from build123d import *

# Parameters (mm, degrees)
F1_DEPTH = 121.92
F3_DEPTH = 60.96
F4_W     = 60.96
F4_H     = 40.64
F5_DEPTH = 121.921


with BuildPart() as f1:
    # F0 (on Front) → F1 (new body)
    with BuildSketch(Plane.XZ):
        Polygon((137.16, -40.64), (137.16, 40.64), (15.24, 40.64), (-137.16, 40.64), (-137.16, -40.64), align=None)
        Polygon((15.24, 40.64), (137.16, 40.64), (137.16, 101.6), (106.68, 101.6), (106.68, 121.92), (45.72, 121.92), (45.72, 101.6), (15.24, 101.6), align=None)
    extrude(amount=F1_DEPTH)

    # F2 (on face) → F3 (cut)
    with BuildSketch(Plane.XY.offset(40.64)):
        Polygon((15.24, -91.111548), (15.24, -30.151548), (-45.72, -30.151548), (-106.68, -30.151548), (-106.68, -91.111548), align=None)
    extrude(amount=-F3_DEPTH, mode=Mode.SUBTRACT)

    # F4 (on face) → F5 (cut, through all)
    with BuildSketch(Plane.XZ.offset(121.92)):
        with Locations((76.2, 60.96)):
            Rectangle(F4_W, F4_H)
    extrude(amount=-F5_DEPTH, mode=Mode.SUBTRACT)


solid = f1.part
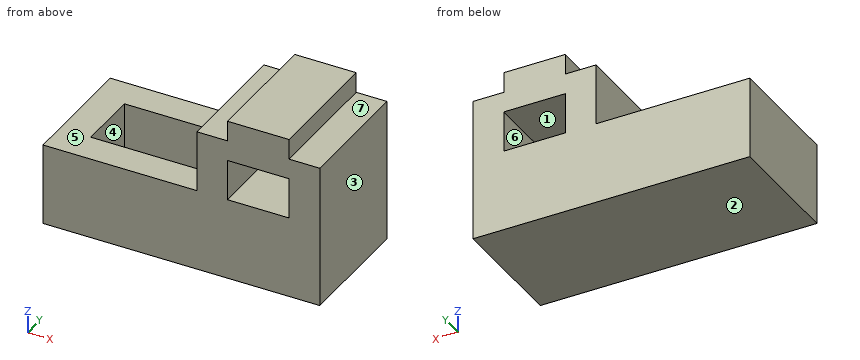
Can you work these out from the model? Positions are in its coordinate system, mm. Face numbers are marked on the shaded views. A direction names the side the tool comes from. Give positions to 0.01 mm unless a question says otherwise; leave off trailing zeros. Order: outer loops, then holes, each group sorted by start corner. A loop starts at its lowest first (then second) coordinate and runs counter-clockwise, first axis right, second up. Notation, with made-up numbers: M 55.25,22 L 72.25,22 A35 ccw 72.25,57 Z; hole C 23,23.5 d8. An arc over 180 degrees is marked long. One line per question, with ' | ' between items.
Item 1: For the marked faces 4, 5, 6 and 7, which set-ups out of +Z, -Z, +X, -X, +Y, -Y let a thin tool reach every point of the face, with its end or its side?
Answer block:
face 4: +Z | face 5: +Z, -X, +Y, -Y | face 6: +Y, -Y | face 7: +Z, +X, +Y, -Y
Item 2: Please list where these lines run through material, in increasing order: L1, parallel to Y at x = -88.5, z = 7; L2, parallel to X at y = -76, z = 67.5; L3, parallel to Z at x = 74, y = -72.
Answer block:
L1: y = -121.92 to -91.11, -30.15 to 0 | L2: x = 15.24 to 45.72, 106.68 to 137.16 | L3: z = -40.64 to 40.64, 81.28 to 121.92
Item 3: Suppose I cut it at B-B, the plane x = 63.5. Write out the boundary of the cut face in (y, z).
Answer block:
outline: M -121.92,-40.64 L 0,-40.64 L 0,40.64 L -121.92,40.64 Z; M -121.92,81.28 L 0,81.28 L 0,121.92 L -121.92,121.92 Z
Item 4: Suppose I cut it at C-C, the plane z = 31.5. Write out the boundary of the cut face in (x, y).
Answer block:
outline: M -137.16,-121.92 L 137.16,-121.92 L 137.16,0 L -137.16,0 Z; hole M -106.68,-91.11 L 15.24,-91.11 L 15.24,-30.15 L -106.68,-30.15 Z
Item 5: We'd pull the mould along X, two halves only. Please class the marked faces 1, 2 and 3: released by +X, released by -X, zero draft, split by the parting line, or undercut.
Answer block:
face 1: undercut | face 2: zero draft | face 3: released by +X
Item 6: Suppose I cut it at A-A, the plane z = 68. Write out the boundary of the cut face in (x, y), then the cut area to 3 significant figures.
Answer block:
outline: M 15.24,-121.92 L 45.72,-121.92 L 45.72,0 L 15.24,0 Z; M 106.68,-121.92 L 137.16,-121.92 L 137.16,0 L 106.68,0 Z | area: 7,430 mm2
Item 7: I'm going to push flat-ended pins straight in: pin 1 Ø15 at (x, y) = (121.5, -54.5) entering from +Z; pin 2 Ø18.5 at (x, y) = (-24.5, -71.5) entering from +Z; pin 3 Ø12 at (y, z) = (-84.5, 71) entering from -X. Where does each tip first touch, or does it pass through?
Answer block:
pin 1: stops at z = 101.6 | pin 2: stops at z = -20.32 | pin 3: stops at x = 15.24
Item 8: Suppose I cut it at D-D, the plane y = -11. Write out the boundary of the cut face in (x, z), then the cut area to 3 significant figures.
Answer block:
outline: M -137.16,-40.64 L 137.16,-40.64 L 137.16,101.6 L 106.68,101.6 L 106.68,121.92 L 45.72,121.92 L 45.72,101.6 L 15.24,101.6 L 15.24,40.64 L -137.16,40.64 Z; hole M 45.72,40.64 L 106.68,40.64 L 106.68,81.28 L 45.72,81.28 Z | area: 28,500 mm2
